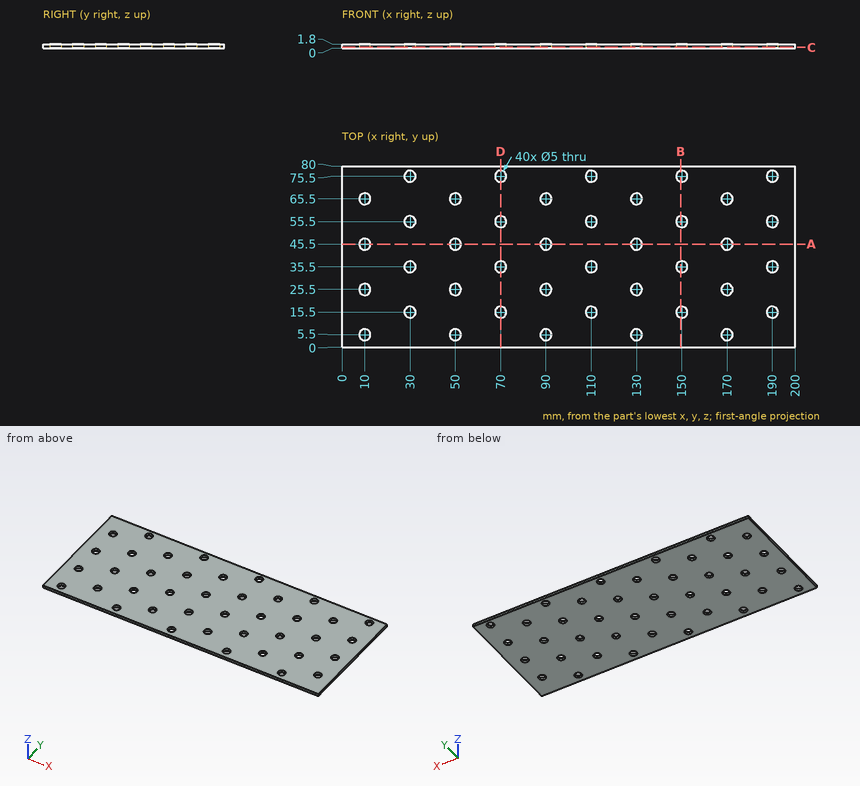
Can you work these out from the drawing? Everything is in mm from the part's minimum corner. Round coordinates to 2 decimals unless told otherwise and drop trailing zeros. Write each loop counter-clockwise with the first axis right and the second up, starting at its lowest first coordinate (ties: lowest second). Pieces come first, ordered by that corner, then holes.
1. Suppose I cut it at C-C (z = 0.35). State how many separate pieces and enclosed holes the cut face has, and give its area (3 significant figures).
2. Suppose I cut it at D-D (x = 70). List the corners of the cut face in (y, z) for me, and give its area (3 significant figures).
3. Suppose I cut it at B-B (x = 149.5). List the corners of the cut face in (y, z) for me.
4. Will this pin go through, and if not, where does the flat tip stop? pin 1 Ø4.5 at (x, y) = (130, 65.5) entering from +Z.
5. I need wall thicknesses on L1, parallel to Y at x = 150, z = 0.4; L2, parallel to Y at x = 10, z = 0.7; L3, parallel to X at y = 56, z = 1.75. Which ranges of each line are inside material? Lowest first, please.
6. Suppose I cut it at A-A (y = 45.5). List the corners of the cut face in (x, z) for me.
Answer sheet:
1. separate pieces: 1
1. enclosed holes: 40
1. area: 15,200 mm2
2. outline: (0, 0) - (13, 0) - (13, 1.8) - (0, 1.8) - close; (18, 0) - (33, 0) - (33, 1.8) - (18, 1.8) - close; (38, 0) - (53, 0) - (53, 1.8) - (38, 1.8) - close; (58, 0) - (73, 0) - (73, 1.8) - (58, 1.8) - close; (78, 0) - (80, 0) - (80, 1.8) - (78, 1.8) - close
2. area: 108 mm2
3. outline: (0, 0) - (13.05, 0) - (13.05, 1.8) - (0, 1.8) - close; (17.95, 0) - (33.05, 0) - (33.05, 1.8) - (17.95, 1.8) - close; (37.95, 0) - (53.05, 0) - (53.05, 1.8) - (37.95, 1.8) - close; (57.95, 0) - (73.05, 0) - (73.05, 1.8) - (57.95, 1.8) - close; (77.95, 0) - (80, 0) - (80, 1.8) - (77.95, 1.8) - close
4. pin 1: passes through
5. L1: y = 0 to 13, 18 to 33, 38 to 53, 58 to 73, 78 to 80
5. L2: y = 0 to 3, 8 to 23, 28 to 43, 48 to 63, 68 to 80
5. L3: x = 0 to 27.55, 32.45 to 67.55, 72.45 to 107.55, 112.45 to 147.55, 152.45 to 187.55, 192.45 to 200
6. outline: (0, 0) - (7.5, 0) - (7.5, 1.8) - (0, 1.8) - close; (12.5, 0) - (47.5, 0) - (47.5, 1.8) - (12.5, 1.8) - close; (52.5, 0) - (87.5, 0) - (87.5, 1.8) - (52.5, 1.8) - close; (92.5, 0) - (127.5, 0) - (127.5, 1.8) - (92.5, 1.8) - close; (132.5, 0) - (167.5, 0) - (167.5, 1.8) - (132.5, 1.8) - close; (172.5, 0) - (200, 0) - (200, 1.8) - (172.5, 1.8) - close
